```python
from build123d import *

# Parameters (mm, degrees)
SKETCH_1_W          = 15
SKETCH_1_H          = 15
SKETCH_1_W_2        = 13
SKETCH_1_H_2        = 13
EXTRUDE_1_DEPTH     = 235
SKETCH_2_R          = 1.5
CUT_EXTRUDE_1_DEPTH = 236.597644301
SKETCH_3_R          = 1.5
CUT_EXTRUDE_2_DEPTH = 236.597644301


with BuildPart() as part:
    # 草图1 → 凸台-拉伸1 (new body)
    with BuildSketch(Plane(origin=(0, 0, 0), x_dir=(1, 0, 0), z_dir=(0, 1, 0))):
        Rectangle(SKETCH_1_W, SKETCH_1_H)
        Rectangle(SKETCH_1_W_2, SKETCH_1_H_2, mode=Mode.SUBTRACT)
    extrude(amount=EXTRUDE_1_DEPTH)

    # 草图2 → 切除-拉伸1 (cut, through all)
    with BuildSketch(Plane.XY.offset(7.5)):
        with Locations((0, 127.5)):
            Circle(SKETCH_2_R)
        with Locations((0, 107.5)):
            Circle(SKETCH_2_R)
        with Locations((0, 151.5)):
            Circle(SKETCH_2_R)
        with Locations((0, 83.5)):
            Circle(SKETCH_2_R)
    extrude(amount=-CUT_EXTRUDE_1_DEPTH, mode=Mode.SUBTRACT)

    # 草图3 → 切除-拉伸2 (cut, through all)
    with BuildSketch(Plane(origin=(7.5, 0, 0), x_dir=(0, 0, -1), z_dir=(1, 0, 0))):
        with Locations((0, 215)):
            Circle(SKETCH_3_R)
        with Locations((0, 20)):
            Circle(SKETCH_3_R)
    extrude(amount=-CUT_EXTRUDE_2_DEPTH, mode=Mode.SUBTRACT)


solid = part.part
```
Can you work these out from the model? Positions are in its coordinate system, mm. A direction names the side the tool comes from. Coordinates: 2 decimals unless noted, no trailing zeros. Loops run counter-clockwise (first coordinate to the right, second up) from the corner with the lowest first, then second, coordinate; pieces in that order, holes last.
Item 1: Suppose I cut it at A-A (z = -3.5). Please give me the cut outline in (x, y), then the cut area to 3 significant figures.
Answers below:
outline: (-7.5, 0) - (-6.5, 0) - (-6.5, 235) - (-7.5, 235) - close; (6.5, 0) - (7.5, 0) - (7.5, 235) - (6.5, 235) - close
area: 470 mm2
Item 2: If we mould it in two halves opening along X, with no side actions, what happens to faces 1 (the face through (-6.5, 116, 0)), 2 (the face through (7.5, 116, 0)), 3 (the face through (0, 116, -7.5)), 4 (the face through (-7.5, 116, 0))? For each: released by +X, released by -X, zero draft, split by the parting line, or undercut.
Answers below:
face 1: undercut
face 2: released by +X
face 3: zero draft
face 4: released by -X
Item 3: Please list where these lines run through material, in increasing order: L1, parallel to Y at x = -7.2, z = 0; L2, parallel to Z at x = 1.5, y = 121; L3, parallel to Y at x = 0, z = 7.
Answers below:
L1: y = 0 to 18.5, 21.5 to 213.5, 216.5 to 235
L2: z = -7.5 to -6.5, 6.5 to 7.5
L3: y = 0 to 82, 85 to 106, 109 to 126, 129 to 150, 153 to 235
Item 4: Suppose I cut it at B-B (y = 102.5). Please give me the cut outline in (x, z).
Answers below:
outline: (-7.5, -7.5) - (7.5, -7.5) - (7.5, 7.5) - (-7.5, 7.5) - close; hole (-6.5, -6.5) - (6.5, -6.5) - (6.5, 6.5) - (-6.5, 6.5) - close
Item 5: I'm going to push a flat-ended pin straight in: pin 1 (3.5 mm diameter, centred on x = 0, y = 107.5, fed in from +Z). Where does the tip first touch, or does it pass through?
Answers below:
pin 1: stops at z = 7.5
Item 6: Which directions (+Z, -Z, +X, -X, +Y, -Y) give clear straight access to the entire face, cutting with the end or side of a thin tool? Please do faces 5 (the face through (6.5, 116, 0)), 6 (the face through (-7, 235, 0)).
Answers below:
face 5: +Y, -Y
face 6: +Z, -Z, +X, -X, +Y
